Verification items for the finished model (mm, model axes). Give positions to 0.01 mm unless a question says otherwise; leave off trailing zeros. Loops run counter-clockwise (first coordinate to the right, second up) from the corner with the lowest first, then second, coordinate; pieces in that order, holes last. Notation, with made-up numbers: (9.5, 36) - (55.5, 36) arc R30 cw to (55.5, 59) - close; hole circle Ø11 at (-14.75, -23.5). An arc over 180 degrees is marked (long way). One line per item, written item: value. Start each with the question number.
1. Scan lines: L1, parallel to X at y = 106.5, z = 7.5; L2, parallel to Y at x = 99, z = 7.5; L3, parallel to Y at x = 254, z = 3.5. Record each from-to range of solid material in increasing order. Write a range as [from, to].
2. Sectioned sample at B-B (x = 254). Record the cut outline in (y, z), plus the area to 3 significant figures.
3. Sectioned sample at C-C (y = 63.5). Record the cut outline in (x, z), plus the area to 3 significant figures.
4. Gauge pin test, flat ends, axial feed: pin 1 (3 mm diameter, centred on y = 87, z = 10, fed in from +X); pin 2 (13.5 mm diameter, centred on x = 254, y = 63.5, fed in from +Z); pin 3 (4 mm diameter, centred on x = 236.5, z = 6, fed in from +Y); pin 4 (6.5 mm diameter, centred on x = 237.5, z = 6, fed in from -Y). Record the tip position at first contact, or that the pin passes through.
5. Sectioned sample at D-D (x = 80.5). Record the cut outline in (y, z).
6. Sectioned sample at A-A (z = 9.75). Count the separate pieces of the cut face and the enclosed holes in it, plus the area to 3 significant figures.
from build123d import *

# Parameters (mm, degrees)
F0_W     = 88.9
F0_H     = 25.4
F1_DEPTH = 12.7
F2_R     = 7.62
F3_DEPTH = 48.26
F5_DEPTH = 6.35
F6_R     = 5.08
F7_R     = 25.4
F8_R     = 10.16


with BuildPart() as f1:
    # F0 (on Top) → F1 (new body)
    with BuildSketch(Plane.XY):
        Polygon((0, 127), (0, 0), (177.8, 0), (177.8, 50.8), (177.8, 76.2), (177.8, 127), align=None)
        with Locations((222.25, 63.5)):
            Rectangle(F0_W, F0_H)
    extrude(amount=F1_DEPTH)

    # F2 (on face) → F3 (cut)
    with BuildSketch(Plane.XY.offset(12.7)):
        with Locations((254, 63.5)):
            Circle(F2_R)
    extrude(amount=-F3_DEPTH, mode=Mode.SUBTRACT)

    # F4 (on face) → F5 (cut)
    with BuildSketch(Plane.XY.offset(12.7)):
        Polygon((171.45, 120.65), (6.35, 120.65), (6.35, 6.35), (171.45, 6.35), (171.45, 50.8), (171.45, 76.2), align=None)
        Polygon((165.1, 12.7), (12.7, 12.7), (12.7, 114.3), (165.1, 114.3), (165.1, 76.2), (165.1, 50.8), align=None, mode=Mode.SUBTRACT)
    extrude(amount=-F5_DEPTH, mode=Mode.SUBTRACT)

    # F6
    f6_edges = [f1.edges().sort_by_distance(p)[0] for p in [
        (6.35, 6.35, 9.525),
        (171.45, 6.35, 9.525),
        (171.45, 120.65, 9.525),
        (6.35, 120.65, 9.525),
        (165.1, 12.7, 9.525),
        (165.1, 114.3, 9.525),
        (12.7, 114.3, 9.525),
        (12.7, 12.7, 9.525),
    ]]
    fillet(f6_edges, radius=F6_R)

    # F7
    f7_edges = [f1.edges().sort_by_distance(p)[0] for p in [
        (177.8, 50.8, 6.35),
        (177.8, 76.2, 6.35),
    ]]
    fillet(f7_edges, radius=F7_R)

    # F8
    f8_edges = [f1.edges().sort_by_distance(p)[0] for p in [
        (266.7, 50.8, 6.35),
        (266.7, 76.2, 6.35),
        (177.8, 0, 6.35),
        (177.8, 127, 6.35),
        (0, 127, 6.35),
        (0, 0, 6.35),
    ]]
    fillet(f8_edges, radius=F8_R)


solid = f1.part
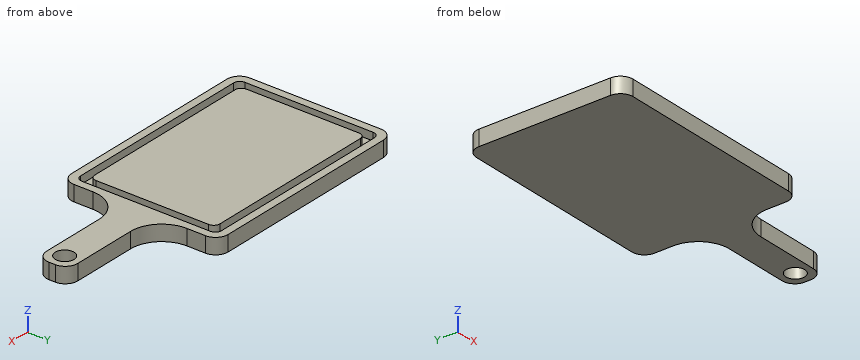
Results are:
1. L1: x = [0, 6.35], [12.7, 165.1], [171.45, 177.8]
1. L2: y = [0, 6.35], [12.7, 114.3], [120.65, 127]
1. L3: y = [50.8, 55.88], [71.12, 76.2]
2. outline: (50.8, 0) - (55.88, 0) - (55.88, 12.7) - (50.8, 12.7) - close; (71.12, 0) - (76.2, 0) - (76.2, 12.7) - (71.12, 12.7) - close
2. area: 129 mm^2
3. outline: (0, 0) - (246.38, 0) - (246.38, 12.7) - (171.45, 12.7) - (171.45, 6.35) - (165.1, 6.35) - (165.1, 12.7) - (12.7, 12.7) - (12.7, 6.35) - (6.35, 6.35) - (6.35, 12.7) - (0, 12.7) - close; (261.62, 0) - (266.7, 0) - (266.7, 12.7) - (261.62, 12.7) - close
3. area: 3,110 mm^2
4. pin 1: stops at x = 183.55
4. pin 2: passes through
4. pin 3: stops at y = 76.2
4. pin 4: stops at y = 50.8
5. outline: (0, 0) - (127, 0) - (127, 12.7) - (120.65, 12.7) - (120.65, 6.35) - (114.3, 6.35) - (114.3, 12.7) - (12.7, 12.7) - (12.7, 6.35) - (6.35, 6.35) - (6.35, 12.7) - (0, 12.7) - close
6. separate pieces: 2
6. enclosed holes: 2
6. area: 21,400 mm^2
